The listing builds one solid part. Answer for the finished solid, in the listing's coordinates (mm). A direction names the side the tool comes from. Coordinates: 2 decimals unless noted, no trailing zeros. Order: outer loops, then holes, each group sorted by start corner. A loop starts at its lowest first (then second) coordinate and runs counter-clockwise, first axis right, second up. Notation, with made-up numbers: M 8.5,71 L 57.5,71 A16 cw 57.5,90 Z; hole C -13.5,63.25 d11. An arc over 180 degrees is marked long. One line per item, written item: value. Start each with the question number.
Q1. Determine the mould class of faces 4 (the cylindrical face through (-4.84, 2.03, 17.82)), 5 (the flat face through (4, -4, 21.535)), 6 (the cylindrical face through (-11.036, -4.289, -5.093)) for opening direction X: pulls with the +X half, pulls with the -X half, needs draft (parallel to the pull), parting line crosses it, or undercut.
Q2. Each of these flat-tipped pins is pushed along its axis until it touches: pin 1 Ø4 at (y, z) = (-0.5, 17) entering from -X; pin 2 Ø4.5 at (x, y) = (1.63, -4.8) entering from +Z; pin 3 Ø2 at (y, z) = (1, 18) entering from -X; pin 4 Ø4.5 at (x, z) = (2.17, 8.78) entering from -Y. Where does it stop, or does it pass through?
Q3. Straight lines are drawn through the part: line 1 along Z through (x, y) = (-2, 1); line 2 along Z through (x, y) = (-4, 3.5); line 3 along X through (y, z) = (2.25, 17). For each, find the intervals that lie inside material, in ascending order. Write a range as [from, to].
Q4. For faces 1 (the cylindrical face through (1.802, 2.028, 10.443)), 2 (the flat face through (-3, 0, 9)), 3 (the cylindrical face through (2.55, -3.37, 23.56)), determine the directions among +Z, -Z, +X, -X, +Y, -Y from which every point of the face is accessible in a straight line to the end or side of a thin tool.
Q5. The part is cut by section B-B on y = -4.8. Give the vertices of the cut face in (x, z).
Q6. The part is cut by section A-A on y = -7. Give the vertices of the cut face in (x, z), then the cut area to 3 significant figures.
Q7. The part is cut by section D-D on x = -14. Give the vertices of the cut face in (y, z).
Q8. The part is cut by section C-C on x = 1. Give the vertices of the cut face in (y, z).
```python
from build123d import *

# Parameters (mm, degrees)
ESTRUSIONE_ESTRUSIONE1_DEPTH = 4
ESTRUSIONE_ESTRUSIONE2_DEPTH = 8
SCHIZZO7_R                   = 1.7
TAGLIO_ESTRUSIONE4_DEPTH     = 13
SCHIZZO10_R                  = 1.7
TAGLIO_ESTRUSIONE5_DEPTH     = 10
SCHIZZO11_R                  = 1.7
TAGLIO_ESTRUSIONE6_DEPTH     = 10


with BuildPart() as part:
    # Schizzo1 → Estrusione-Estrusione1 (new body)
    with BuildSketch(Plane(origin=(0, 0, 0), x_dir=(1, 0, 0), z_dir=(0, 1, 0))):
        Polygon((1.585961517, 7.064649843), (22.133260635, -25.535350157), (-7.866739365, -25.535350157), (-28.414038483, 7.064649843), align=None)
    extrude(amount=ESTRUSIONE_ESTRUSIONE1_DEPTH)

    # Schizzo4 → Estrusione-Estrusione2 (add)
    with BuildSketch(Plane.XZ):
        Polygon((-28.414038483, -7.064649843), (-25.892897487, -3.064649843), (4.107102513, -3.064649843), (1.585961517, -7.064649843), align=None)
        Polygon((22.133260635, 25.535350157), (-7.866739365, 25.535350157), (-10.387880361, 21.535350157), (19.612119639, 21.535350157), align=None)
    extrude(amount=ESTRUSIONE_ESTRUSIONE2_DEPTH)

    # Schizzo7 → Taglio-Estrusione4 (cut, through all)
    with BuildSketch(Plane(origin=(0, 4, 0), x_dir=(1, 0, 0), z_dir=(0, 1, 0))):
        with Locations((7.329259334, -16.787762722)):
            Circle(SCHIZZO7_R)
        with Locations((-3.487605714, -16.787762722)):
            Circle(SCHIZZO7_R)
        with Locations((-8.711706468, -8.681963492)):
            Circle(SCHIZZO7_R)
        with Locations((-13.935807222, -0.576164263)):
            Circle(SCHIZZO7_R)
        with Locations((-2.9886387, -0.77834524)):
            Circle(SCHIZZO7_R)
        with Locations((2.170310317, -8.783053981)):
            Circle(SCHIZZO7_R)
    extrude(amount=-TAGLIO_ESTRUSIONE4_DEPTH, mode=Mode.SUBTRACT)

    # Schizzo10 → Taglio-Estrusione5 (cut)
    with BuildSketch(Plane.XY.offset(25.535350157)):
        with Locations((1.633260635, -4.8)):
            Circle(SCHIZZO10_R)
        with Locations((11.633260635, -4.8)):
            Circle(SCHIZZO10_R)
    extrude(amount=-TAGLIO_ESTRUSIONE5_DEPTH, mode=Mode.SUBTRACT)

    # Schizzo11 → Taglio-Estrusione6 (cut)
    with BuildSketch(Plane(origin=(0, 0, -7.064649843), x_dir=(-1, 0, 0), z_dir=(0, 0, -1))):
        with Locations((9.414038483, -4.8)):
            Circle(SCHIZZO11_R)
        with Locations((19.414038483, -4.8)):
            Circle(SCHIZZO11_R)
    extrude(amount=-TAGLIO_ESTRUSIONE6_DEPTH, mode=Mode.SUBTRACT)


solid = part.part
```
Output:
1. face 4: undercut
1. face 5: needs draft
1. face 6: undercut
2. pin 1: stops at x = -14.47
2. pin 2: stops at z = 25.54
2. pin 3: stops at x = -13.25
2. pin 4: stops at y = 0
3. line 1: z = [-7.06, -0.6], [2.16, 15.96], [17.61, 25.54]
3. line 2: z = [-7.06, -0.59], [2.14, 15.17], [18.41, 25.54]
3. line 3: x = [-13.25, -5.17], [-1.8, 5.64], [9.02, 16.75]
4. face 1: +Y, -Y
4. face 2: +X, -X, -Y
4. face 3: +Z
5. outline: M -28.41,-7.06 L -21.11,-7.06 L -21.11,-3.06 L -25.89,-3.06 Z; M -17.71,-7.06 L -11.11,-7.06 L -11.11,-3.06 L -17.71,-3.06 Z; M -10.39,21.54 L -0.07,21.54 L -0.07,25.54 L -7.87,25.54 Z; M -7.71,-7.06 L 1.59,-7.06 L 4.11,-3.06 L -7.71,-3.06 Z; M 3.33,21.54 L 9.93,21.54 L 9.93,25.54 L 3.33,25.54 Z; M 13.33,21.54 L 19.61,21.54 L 22.13,25.54 L 13.33,25.54 Z
6. outline: M -28.41,-7.06 L 1.59,-7.06 L 4.11,-3.06 L -25.89,-3.06 Z; M -10.39,21.54 L 19.61,21.54 L 22.13,25.54 L -7.87,25.54 Z
6. area: 240 mm^2
7. outline: M -8,-7.06 L 4,-7.06 L 4,-1.12 L 0,-1.12 L 0,-3.06 L -8,-3.06 Z; M 0,2.27 L 4,2.27 L 4,15.8 L 0,15.8 Z
8. outline: M -8,-7.06 L 4,-7.06 L 4,7.55 L 0,7.55 L 0,-3.06 L -8,-3.06 Z; M -8,21.54 L -6.38,21.54 L -6.38,25.54 L -8,25.54 Z; M -3.22,21.54 L 0,21.54 L 0,10.02 L 4,10.02 L 4,25.54 L -3.22,25.54 Z
